Autodesk Inventor part; units mm, degrees
ref_plane "YZ Plane" through (0, 0, 0) normal (1, 0, 0) x (0, 1, 0)
ref_plane "XZ Plane" through (0, 0, 0) normal (0, 1, 0) x (-1, 0, 0)
ref_plane "XY Plane" through (0, 0, 0) normal (0, 0, 1) x (1, 0, 0)
sketch "Sketch1" plane through (0, 0, 0) normal (0, 0, 1) x (1, 0, 0)
  line L0 (-22.25, 17.75) -> (-22.25, 14.75)
  line L1 (-22.25, 14.75) -> (-10.25, 14.75)
  line L2 (-10.25, 14.75) -> (-10.25, 0)
  arc A0 (-10.25, 0) -> (10.25, 0) centre (0, 0) ccw
  line L3 (10.25, 0) -> (10.25, 14.75)
  line L4 (10.25, 14.75) -> (22.25, 14.75)
  line L5 (22.25, 14.75) -> (22.25, 17.75)
  line L6 (22.25, 17.75) -> (-22.25, 17.75)
  point P0 (0, 17.75)
  dimension "d0" = 44.5
  dimension "d1" = 10.25
  dimension "d2" = 3
  dimension "d3" = 17.75
extrude "Extrusion1" add sketch "Sketch1" along normal mid plane 26.5
sketch "Sketch2" plane through (0, 0, 13.25) normal (0, 0, 1) x (1, 0, 0)
  line L0 (-22.25, 17.75) -> (-22.25, 14.75) construction
  line L1 (-22.25, 14.75) -> (-10.25, 14.75) construction
  line L2 (-10.25, 14.75) -> (-10.25, 0) construction
  arc A0 (-10.25, 0) -> (10.25, 0) centre (0, 0) ccw construction
  line L3 (10.25, 0) -> (10.25, 14.75) construction
  line L4 (10.25, 14.75) -> (22.25, 14.75) construction
  line L5 (22.25, 14.75) -> (22.25, 17.75) construction
  line L6 (22.25, 17.75) -> (-22.25, 17.75) construction
  line L7 (-7.75, 17.75) -> (7.75, 17.75)
  line L8 (7.75, 17.75) -> (7.75, 9.1962)
  arc A1 (5.75, 5.1962) -> (7.75, 9.1962) centre (2.75, 9.1962) ccw
  line L9 (5.75, 5.1962) -> (6.5855, 1.4811)
  arc A2 (-6.5855, 1.4811) -> (6.5855, 1.4811) centre (0, 0) ccw
  line L10 (-6.5855, 1.4811) -> (-5.75, 5.1962)
  arc A3 (-7.75, 9.1962) -> (-5.75, 5.1962) centre (-2.75, 9.1962) ccw
  line L11 (-7.75, 9.1962) -> (-7.75, 17.75)
  line L12 (22.25, 17.75) -> (-22.25, 17.75)
  point P0 (0, 17.75)
  dimension "d6" = 5
  dimension "d7" = 6.75
  dimension "d8" = 2.5
  dimension "d9" = 11.5
  dimension "d10" = 7.75
extrude "Extrusion2" cut sketch "Sketch2" against normal blind 26.5
sketch "Sketch3" plane through (0, 0, 0) normal (0, 0, 1) x (1, 0, 0)
  circle A0 centre (0, 0) radius 7.75
  dimension "d13" = 15.5
extrude "Extrusion3" cut sketch "Sketch3" along normal mid plane 24
sketch "Sketch4" plane through (-22.25, 17.75, 13.25) normal (0, 1, 0) x (1, 0, 0)
  line L0 (0, 26.5) -> (14.5, 26.5)
  line L1 (44.5, 26.5) -> (44.5, 0)
  point P0 (22.25, 13.25)
  point P1 (0, 0)
  point P2 (6.25, 13.25)
  point P3 (38.25, 13.25)
  dimension "d16" = 6.25
  dimension "d17" = 13.25
  dimension "d19" = 6.25
hole "Hole1" at (-16, 17.75, 0) at (16, 17.75, 0) direction (0, -1, 0) diameter 3.2 end through all
properties part number "Heated Bed Bearing Mount"
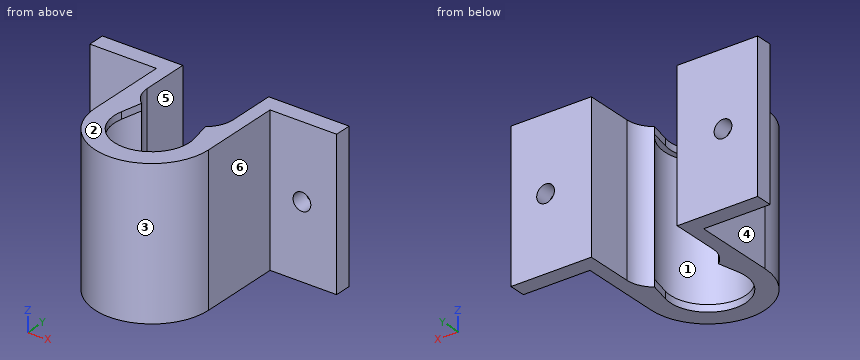
Verification items for the finished model (mm, model axes). Face numbers are marked on the shaded views. A direction names the side the tool comes from. Coordinates: 2 decimals unless noted, no trailing zeros. Write each loop counter-clockwise with the first axis right and the second up, starting at its lowest first coordinate (ties: lowest second). Pieces come first, ordered by that corner, then holes. Notation, with made-up numbers: M 29,-18.75 L 41,-18.75 A38 cw 41,19.25 Z; hole C 83.5,64.5 d8. An arc over 180 degrees is marked long. Use a Markdown table: item, result.
Q1. Go/stop test with flat-tipped pins: P1, Ø12, axis at x = 17, z = 6.5, coming from the -Y side; P2, Ø13, axis at x = -14, z = 5.5, coming from the -Y side; P3, Ø12, axis at y = 2.5, z = 10, coming from the -X side. Record where each tip stops, or that it passes through.
Reply:
| item | result |
|---|---|
| P1 | stops at y = 14.75 |
| P2 | stops at y = -6.99 |
| P3 | stops at x = -10.25 |
Q2. Sectioned sample at B-B, the plane x = 16. Record the boundary of the cut face in (y, z).
Reply:
| item | result |
|---|---|
| outline | M 14.75,-13.25 L 17.75,-13.25 L 17.75,-1.6 L 14.75,-1.6 Z; M 14.75,1.6 L 17.75,1.6 L 17.75,13.25 L 14.75,13.25 Z |
Q3. Thickness scan on line 1 (X direction, y = 16.9, z = 0); line 2 (Z direction, x = -16, y = 16.75); line 3 (X direction, y = 11, z = -4.25). Record the ranges inside material, lowest first.
Reply:
| item | result |
|---|---|
| line 1 | x = -22.25 to -17.6, -14.4 to -7.75, 7.75 to 14.4, 17.6 to 22.25 |
| line 2 | z = -13.25 to -1.6, 1.6 to 13.25 |
| line 3 | x = -10.25 to -7.75, 7.75 to 10.25 |
Q4. Sectioned sample at A-A, the plane y = 15.5. Record the boundary of the cut face in (x, z), plus the area to 3 significant figures.
Reply:
| item | result |
|---|---|
| outline | M -22.25,-13.25 L -7.75,-13.25 L -7.75,13.25 L -22.25,13.25 Z; M 7.75,-13.25 L 22.25,-13.25 L 22.25,13.25 L 7.75,13.25 Z; hole C -16,0 d3.2; hole C 16,0 d3.2 |
| area | 752 mm² |
Q5. Sectioned sample at C-C, the plane y = 0.75. Record the boundary of the cut face in (x, z), plus the area to 3 significant figures.
Reply:
| item | result |
|---|---|
| outline | M -10.25,-13.25 L -6.71,-13.25 L -6.71,-12 L -7.71,-12 L -7.71,12 L -6.71,12 L -6.71,13.25 L -10.25,13.25 Z; M 6.71,-13.25 L 10.25,-13.25 L 10.25,13.25 L 6.71,13.25 L 6.71,12 L 7.71,12 L 7.71,-12 L 6.71,-12 Z |
| area | 139 mm² |
Q6. Sectioned sample at D-D, the plane z = 0. Count the separate pieces of the cut face and the enclosed holes in it, plus the area to 3 significant figures.
Reply:
| item | result |
|---|---|
| separate pieces | 3 |
| enclosed holes | 0 |
| area | 224 mm² |
Q7. Draft check along X on the marked faces 1, 2 and 3. Enter one of: +X half, -X half, draft (parallel to the pull), parting line (faces both ways), or undercut.
Reply:
| item | result |
|---|---|
| face 1 | undercut |
| face 2 | draft |
| face 3 | parting line |
Q8. Set-up check for the marked faces 4, 5 and 6: record each of +Z, -Z, +X, -X, +Y, -Y from which the full face is reachable in a straight line by a thin tool's end or side.
Reply:
| item | result |
|---|---|
| face 4 | +Z, -Z, -X, -Y |
| face 5 | +Z, -Z, +Y |
| face 6 | +Z, -Z, +X, -Y |
